from build123d import *

# Parameters (mm, degrees)
SKETCH2_W                 = 304.8
SKETCH2_H                 = 101.6
SKETCH2_R                 = 6.35
SKETCH2_R_2               = 7
BOSS_EXTRUDE1_DEPTH       = 20
SKETCH3_R                 = 3.25
CUT_EXTRUDE1_DEPTH        = 162.883909021
CIRPATTERN1_COUNT         = 4
LPATTERN1_COUNT           = 2
LPATTERN1_PITCH           = 152.4
LPATTERN1_COPY_1_SKETCH_R = 3.25
LPATTERN1_COPY_1_DEPTH    = 162.883909021
LPATTERN1_COPY_2_SKETCH_R = 3.25
LPATTERN1_COPY_2_DEPTH    = 162.883909021
LPATTERN1_COPY_3_SKETCH_R = 3.25
LPATTERN1_COPY_3_DEPTH    = 162.883909021


with BuildPart() as part:
    # Sketch2 → Boss-Extrude1 (new body)
    with BuildSketch(Plane(origin=(0, 0, 0), x_dir=(1, 0, 0), z_dir=(0, 1, 0))):
        Rectangle(SKETCH2_W, SKETCH2_H)
        with Locations(Location((0, 0, 0), (0, 0, 270))):
            Circle(SKETCH2_R, mode=Mode.SUBTRACT)
        with Locations(Location((-76.2, 0, 0), (0, 0, 270))):
            Circle(SKETCH2_R_2, mode=Mode.SUBTRACT)
        with Locations(Location((76.2, 0, 0), (0, 0, 270))):
            Circle(SKETCH2_R_2, mode=Mode.SUBTRACT)
    extrude(amount=BOSS_EXTRUDE1_DEPTH)

    # Sketch3 → Cut-Extrude1 (cut, through all)
    with BuildSketch(Plane(origin=(0, 20, 0), x_dir=(1, 0, 0), z_dir=(0, 1, 0))):
        with Locations(Location((-76.2, 19, 0), (0, 0, 270))):
            Circle(SKETCH3_R)
    cut_extrude1 = extrude(amount=-CUT_EXTRUDE1_DEPTH, mode=Mode.SUBTRACT)

    # CirPattern1: Cut-Extrude1 ×4 about axis
    cirpattern1_axis = Axis((-76.2, 0, 0), (0, 1, 0))
    for i in range(1, CIRPATTERN1_COUNT):
        add(cut_extrude1.rotate(cirpattern1_axis, i * 360 / CIRPATTERN1_COUNT), mode=Mode.SUBTRACT)

    # LPattern1: Cut-Extrude1 ×2
    with Locations(*[(i * LPATTERN1_PITCH, 0, 0) for i in range(1, LPATTERN1_COUNT)]):
        add(cut_extrude1, mode=Mode.SUBTRACT)

    # LPattern1 copy 1 sketch → LPattern1 copy 1 (cut, through all)
    with BuildSketch(Plane(origin=(76.2, 20, -76.2), x_dir=(0, 0, -1), z_dir=(0, 1, 0))):
        with Locations(Location((-76.2, 19, 0), (0, 0, 270))):
            Circle(LPATTERN1_COPY_1_SKETCH_R)
    extrude(amount=-LPATTERN1_COPY_1_DEPTH, mode=Mode.SUBTRACT)

    # LPattern1 copy 2 sketch → LPattern1 copy 2 (cut, through all)
    with BuildSketch(Plane(origin=(0, 20, 0), x_dir=(-1, 0, 0), z_dir=(0, 1, 0))):
        with Locations(Location((-76.2, 19, 0), (0, 0, 270))):
            Circle(LPATTERN1_COPY_2_SKETCH_R)
    extrude(amount=-LPATTERN1_COPY_2_DEPTH, mode=Mode.SUBTRACT)

    # LPattern1 copy 3 sketch → LPattern1 copy 3 (cut, through all)
    with BuildSketch(Plane(origin=(76.2, 20, 76.2), x_dir=(0, 0, 1), z_dir=(0, 1, 0))):
        with Locations(Location((-76.2, 19, 0), (0, 0, 270))):
            Circle(LPATTERN1_COPY_3_SKETCH_R)
    extrude(amount=-LPATTERN1_COPY_3_DEPTH, mode=Mode.SUBTRACT)


solid = part.part
Read the model definition and answer for the solid it produces. Units are mm, in the model's axes. Give positions to 0.01 mm unless a question says otherwise; leave off trailing zeros. Write each loop counter-clockwise with the first axis right and the second up, starting at its lowest first coordinate (ties: lowest second). Pieces come first, ordered by that corner, then holes. Notation, with made-up numbers: (-1.75, 37) - (37.25, 37) arc R22 ccw to (37.25, 56) - close; hole circle Ø7 at (-0.75, -18.75). An arc over 180 degrees is marked (long way). Answer in a Markdown table with one row per item. Add a question column.
Item 1: Determine the mould class of faces 1 (the face through (-2, 10, -50.8)), 2 (the face through (-79.373, 10.14, -19.705)), 3 (the face through (-152.4, 10, 1)) for opening direction Z: pulls with the +Z half, pulls with the -Z half, needs draft (parallel to the pull), parting line crosses it, or undercut.
Item 2: Section A-A, the plane z = 0 is taken. Count the separate pieces of the cut face and the enclosed holes in it, and give its area (3 significant figures).
Item 3: Section B-B, the plane x = 0 is taken. Write down the section's boundary in (y, z).
Item 4: A flat-ended cylindrical pin translates along its axis: P1, Ø5, axis at x = -76.2, z = -19, coming from the -Y side. Find the tip coordinate at first contact, or state that the pin passes through.
Item 5: Find the intervals of material crossed by L1, parallel to X at y = 4.75, z = -19; L2, parallel to Z at x = 95.2, y = 14.75; L3, parallel to X at y = 3.75, z = -5.5, in increasing order.
Item 6: Section D-D, the plane x = 76.2 is taken. Write down the section's boundary in (y, z), and give its area (3 significant figures).
Recorded:
| question | item | result |
|---|---|---|
| 1 | face 1 | pulls with the -Z half |
| 1 | face 2 | undercut |
| 1 | face 3 | needs draft |
| 2 | separate pieces | 8 |
| 2 | enclosed holes | 0 |
| 2 | area | 4,760 mm2 |
| 3 | outline | (0, -50.8) - (20, -50.8) - (20, -6.35) - (0, -6.35) - close; (0, 6.35) - (20, 6.35) - (20, 50.8) - (0, 50.8) - close |
| 4 | P1 | passes through |
| 5 | L1 | x = -152.4 to -79.45, -72.95 to 72.95, 79.45 to 152.4 |
| 5 | L2 | z = -50.8 to -3.25, 3.25 to 50.8 |
| 5 | L3 | x = -152.4 to -80.53, -71.87 to -3.17, 3.17 to 71.87, 80.53 to 152.4 |
| 6 | outline | (0, -50.8) - (20, -50.8) - (20, -22.25) - (0, -22.25) - close; (0, -15.75) - (20, -15.75) - (20, -7) - (0, -7) - close; (0, 7) - (20, 7) - (20, 15.75) - (0, 15.75) - close; (0, 22.25) - (20, 22.25) - (20, 50.8) - (0, 50.8) - close |
| 6 | area | 1,490 mm2 |
